```python
from build123d import *

# Parameters (mm, degrees)
EXTRUDE_1_DEPTH           = 15
SKETCH_2_R                = 40.75
CUT_EXTRUDE_1_DEPTH       = 8
SKETCH_3_R                = 35.5
CUT_EXTRUDE_2_DEPTH       = 6
SKETCH_4_R                = 33
CUT_EXTRUDE_3_DEPTH       = 203.98029461
CHAMFER_1_SIZE            = 1
FILLET_1_R                = 4.5
FILLET_2_R                = 3
HOLE_WIZARD_1_OUTLINE_R   = 7
HOLE_WIZARD_1_DEPTH       = 10
HOLE_START                = 10
HOLE_WIZARD_1_2_OUTLINE_R = 3
HOLE_WIZARD_1_2_DEPTH     = 5


# Read off the part's stored shape, not the designer's step: 孔1
with BuildPart() as part:
    # 草图1 → 凸台-拉伸1 (new body)
    with BuildSketch(Plane.XY):
        with BuildLine():
            Line((76, 0), (76, -112))
            ThreePointArc((76, -112), (0, -188), (-76, -112))
            Line((-76, -112), (-76, 0))
            ThreePointArc((-76, 0), (0, 76), (76, 0))
        make_face()
    extrude(amount=EXTRUDE_1_DEPTH)

    # 草图2 → 切除-拉伸1 (cut)
    with BuildSketch(Plane.XY.offset(15)):
        with BuildLine():
            Line((50.5, 0), (50.5, -112))
            ThreePointArc((50.5, -112), (0, -162.5), (-50.5, -112))
            Line((-50.5, -112), (-50.5, 0))
            ThreePointArc((-50.5, 0), (0, 50.5), (50.5, 0))
        make_face()
        Circle(SKETCH_2_R, mode=Mode.SUBTRACT)
    extrude(amount=-CUT_EXTRUDE_1_DEPTH, mode=Mode.SUBTRACT)

    # 草图3 → 切除-拉伸2 (cut)
    with BuildSketch(Plane.XY.offset(15)):
        Circle(SKETCH_3_R)
    extrude(amount=-CUT_EXTRUDE_2_DEPTH, mode=Mode.SUBTRACT)

    # 草图4 → 切除-拉伸3 (cut, through all)
    with BuildSketch(Plane.XY.offset(9)):
        Circle(SKETCH_4_R)
    extrude(amount=-CUT_EXTRUDE_3_DEPTH, mode=Mode.SUBTRACT)

    # 倒角1
    chamfer_1_edges = [part.edges().sort_by_distance(p)[0] for p in [
        (-33, 0, 0),
        (-33, 0, 9),
    ]]
    chamfer(chamfer_1_edges, length=CHAMFER_1_SIZE)

    # 圆角1
    fillet_1_edges = [part.edges().sort_by_distance(p)[0] for p in [
        (0, 50.5, 7),
        (50.5, -56, 7),
        (0, -162.5, 7),
        (-50.5, -56, 7),
        (-40.75, 0, 7),
    ]]
    fillet(fillet_1_edges, radius=FILLET_1_R)

    # 圆角2
    fillet_2_edges = [part.edges().sort_by_distance(p)[0] for p in [
        (76, -56, 0),
        (0, -188, 0),
        (-76, -56, 0),
        (0, 76, 0),
    ]]
    fillet(fillet_2_edges, radius=FILLET_2_R)

    # 孔1 outline → 孔1 (cut)
    with BuildSketch(Plane.XY):
        with Locations((0, 65)):
            Circle(HOLE_WIZARD_1_OUTLINE_R)
        with Locations((0, -177)):
            Circle(HOLE_WIZARD_1_OUTLINE_R)
        with Locations((-65, -112)):
            Circle(HOLE_WIZARD_1_OUTLINE_R)
        with Locations((-65, 0)):
            Circle(HOLE_WIZARD_1_OUTLINE_R)
        with Locations((65, -112)):
            Circle(HOLE_WIZARD_1_OUTLINE_R)
        with Locations((65, 0)):
            Circle(HOLE_WIZARD_1_OUTLINE_R)
    extrude(amount=HOLE_WIZARD_1_DEPTH, mode=Mode.SUBTRACT)

    # Hole Wizard 1 2 outline → Hole Wizard 1 2 (cut)
    with BuildSketch(Plane.XY.offset(HOLE_START)):
        with Locations((0, 65)):
            Circle(HOLE_WIZARD_1_2_OUTLINE_R)
        with Locations((0, -177)):
            Circle(HOLE_WIZARD_1_2_OUTLINE_R)
        with Locations((-65, -112)):
            Circle(HOLE_WIZARD_1_2_OUTLINE_R)
        with Locations((-65, 0)):
            Circle(HOLE_WIZARD_1_2_OUTLINE_R)
        with Locations((65, -112)):
            Circle(HOLE_WIZARD_1_2_OUTLINE_R)
        with Locations((65, 0)):
            Circle(HOLE_WIZARD_1_2_OUTLINE_R)
    extrude(amount=HOLE_WIZARD_1_2_DEPTH, mode=Mode.SUBTRACT)


solid = part.part
```
Geometry: final body of the model. Coordinates: model frame, mm. A direction names the side the tool comes from. Coordinates: 2 decimals unless noted, no trailing zeros.
Item 1: Section query A-A (x = 0). State how many separate pieces and enclosed holes the cut face has, then the cut area to 3 significant figures.
Answer:
separate pieces: 4
enclosed holes: 0
area: 1,560 mm2
Item 2: Material intervals for line 1 along Y through (x, z) = (0, 6.75); line 2 along Y through (x, z) = (65, 3.25); line 3 along Y through (x, z) = (30, 13.75), sorted ascending.
Answer:
line 1: y = -188 to -184, -170 to -33, 33 to 58, 72 to 76
line 2: y = -151.38 to -119, -105 to -7, 7 to 39.38
line 3: y = -181.83 to -152.62, -27.58 to -18.98, 18.98 to 27.58, 40.62 to 69.83
Item 3: Draft query along X for faces 1 (the face through (-1.67, 75.98, 8.92)), 2 (the face through (-1.11, 50.488, 13.274)), 3 (the face through (52, -54, 15)), 4 (the face through (-1.517, -183.834, 4.93)). Return one class per face: released by +X, released by -X, zero draft, split by the parting line, or undercut.
Answer:
face 1: split by the parting line
face 2: undercut
face 3: zero draft
face 4: undercut
Item 4: Access query for faces 5 (the face through (1.11, -162.488, 13.274)), 6 (the face through (-64, -115, 10)), 7 (the face through (62, 0, 12)). Directions: +Z, -Z, +X, -X, +Y, -Y. A direction counts if a zero-diameter tool reaches every point of the face in a straight line with its end or side. Return the directions, or none.
Answer:
face 5: +Z
face 6: -Z
face 7: +Z, -Z
Item 5: Contact query for flat-ended pins moving along their axis: P1, Ø6, axis at y = -132.5, z = 6.5, coming from the -X side; P2, Ø22.5, axis at x = 0, y = 65, coming from the +Z side; P3, Ø5, axis at x = 65, y = 0, coming from the +Z side; P4, Ø7, axis at x = 0, y = -177, coming from the -Z side. Output: stop coordinate, or through.
Answer:
P1: stops at x = -73.96
P2: stops at z = 15
P3: passes through
P4: stops at z = 10
